Autodesk Inventor part; units mm, degrees
ref_plane "YZ Plane" through (0, 0, 0) normal (1, 0, 0) x (0, 1, 0)
ref_plane "XZ Plane" through (0, 0, 0) normal (0, 1, 0) x (-1, 0, 0)
ref_plane "XY Plane" through (0, 0, 0) normal (0, 0, 1) x (1, 0, 0)
sketch "Sketch1" plane through (0, 0, 0) normal (0, 0, 1) x (1, 0, 0)
  line L0 (0, 0) -> (110, 0)
  line L1 (110, 0) -> (110, 73)
  line L2 (110, 73) -> (0, 73)
  line L3 (6, 57) -> (50, 57)
  line L4 (50, 57) -> (50, 27)
  line L5 (6, 57) -> (0, 57)
  line L6 (0, 73) -> (0, 57)
  line L7 (0, 27) -> (0, 0)
  line L8 (0, 27) -> (50, 27)
  dimension "d0" = 110
  dimension "d2" = 16
  dimension "d19" = 57
  dimension "d22" = 50
  dimension "d66" = 30
extrude "Extrusion1" add sketch "Sketch1" along normal blind 6
sketch "Sketch2" plane through (0, 0, 6) normal (0, 0, 1) x (1, 0, 0)
  line L0 (105, 0) -> (105, 5)
  line L1 (105, 5) -> (5, 5)
  line L2 (5, 5) -> (5, 0)
  line L3 (0, 27) -> (0, 0)
  line L4 (0, 0) -> (110, 0)
  dimension "d13" = 100
  dimension "d14" = 5
  dimension "d15" = 5
extrude "Extrusion2" cut sketch "Sketch2" against normal blind 10
sketch "Sketch3" plane through (0, 0, 0) normal (0, 0, -1) x (-1, 0, 0)
  line L0 (-331.8351, -68) -> (-331.8351, 72) construction
  line L1 (218.6881, -67.4159) -> (-331.3119, -67.4159)
  line L2 (-331.8351, 72) -> (218.1649, 72)
  line L3 (-50.021, 72.5841) -> (-50.021, -67.4159)
  line L4 (-301.8351, 60.0199) -> (-301.8351, -95.3329) construction
  line L5 (-194.8351, 50.8275) -> (-194.8351, -92.5752) construction
  line L6 (-289.8351, 60.0199) -> (-289.8351, -99.0099) construction
  line L7 (-182.8351, -92.5752) -> (-182.8351, 81.6223) construction
  line L8 (-224.6619, -78.1083) -> (-224.6619, -12.2159) construction
  line L9 (-184.2519, -76.0321) -> (-184.2519, -10.2421) construction
  line L10 (-223.8335, -61.4159) -> (-147.922, -61.4159) construction
  line L11 (-179.8519, -67.4159) -> (-179.8519, -42.4159) construction
  line L12 (-229.1619, -42.4159) -> (-229.1619, -67.4159) construction
  line L13 (-73.021, 109.947) -> (-73.021, -118.6448) construction
  line L14 (-147.521, 95.654) -> (-147.521, -118.6448) construction
  line L15 (-208.521, 101.2387) -> (-208.521, -106.3335) construction
  line L16 (-237.7385, -71.614) -> (-237.7385, -46.614)
  line L17 (243.9615, -46.614) -> (243.9615, -71.614)
  line L18 (-92.021, 52) -> (-57.021, 52) construction
  line L19 (-57.021, 52) -> (-57.021, 27) construction
  line L20 (-57.021, 27) -> (-92.021, 27) construction
  line L21 (-92.021, 27) -> (-92.021, 52) construction
  line L22 (-301.8351, 2.5165) -> (201.7932, 2.5165) construction
  line L23 (-105, 0) -> (-105, 5)
  line L24 (-105, 5) -> (-5, 5)
  line L25 (-5, 5) -> (-5, 0)
  line L26 (0, 0) -> (-5, 0)
  line L27 (0, 27) -> (0, 0)
  line L28 (-50, 27) -> (0, 27)
  line L29 (-50, 57) -> (-50, 27)
  line L30 (0, 57) -> (-50, 57)
  line L31 (0, 73) -> (0, 57)
  line L32 (-110, 73) -> (0, 73)
  line L33 (-110, 0) -> (-110, 73)
  line L34 (-105, 0) -> (-110, 0)
  point P0 (-53.9258, 1.4801)
  point P1 (-331.3119, -67.4159)
  point P2 (-266.7948, -13.3199)
  point P3 (-301.8351, 60.0199)
  point P4 (-301.8351, -95.3329)
  point P5 (-289.8351, 2.5165)
  point P6 (-194.8351, 2.5165)
  point P7 (-182.8351, 2.5165)
  point P8 (189.7932, 2.5165)
  point P9 (94.7932, 2.5165)
  point P10 (82.7932, 2.5165)
  point P11 (-50.021, -58.9159)
  point P12 (-224.6619, -61.4159)
  point P13 (-184.2519, -61.4159)
  point P14 (124.6199, -61.4159)
  point P15 (84.2099, -61.4159)
  point P16 (-73.021, 12.3841)
  point P17 (-27.021, 12.3841)
  point P18 (-319.3351, 69)
  point P19 (-261.0351, 69)
  point P20 (-202.7351, 69)
  point P21 (-144.4351, 69)
  point P22 (-86.1351, 69)
  point P23 (-27.8351, 69)
  point P24 (30.4649, 69)
  point P25 (88.7649, 69)
  point P26 (147.0649, 69)
  point P27 (205.3649, 69)
  point P28 (-325.3351, 62)
  point P29 (-325.3351, 54)
  point P30 (-325.3351, 46)
  point P31 (-325.3351, 38)
  point P32 (-325.3351, 30)
  point P33 (-325.3351, 22)
  point P34 (-325.3351, 14)
  point P35 (-325.3351, 6)
  point P36 (-325.3351, -2)
  point P37 (-325.3351, -10)
  point P38 (-325.3351, -18)
  point P39 (-325.3351, -26)
  point P40 (-325.3351, -34)
  point P41 (225.2932, -34)
  point P42 (225.2932, -26)
  point P43 (225.2932, -18)
  point P44 (225.2932, -10)
  point P45 (225.2932, -2)
  point P46 (225.2932, 6)
  point P47 (225.2932, 14)
  point P48 (225.2932, 22)
  point P49 (225.2932, 30)
  point P50 (225.2932, 38)
  point P51 (225.2932, 46)
  point P52 (225.2932, 54)
  point P53 (225.2932, 62)
  point P54 (-242.2385, -65.614)
  point P55 (248.4615, -65.614)
  dimension "d32" = 30
  dimension "d33" = 12
  dimension "d34" = 137
  dimension "d35" = 12
  dimension "d36" = 8.5
  dimension "d37" = 4.4
  dimension "d38" = 4.5
  dimension "d39" = 6
  dimension "d40" = 23
  dimension "d41" = 97.5
  dimension "d42" = 158.5
  dimension "d43" = 3
  dimension "d44" = 12.5
  dimension "d45" = 58.3
  dimension "d46" = 6.5
  dimension "d47" = 10
  dimension "d48" = 8
  dimension "d49" = 35
  dimension "d50" = 35
  dimension "d51" = 25
  dimension "d52" = 4.5
  dimension "d53" = 4.5
  dimension "d56" = 20
  dimension "d57" = 7
  dimension "d58" = 1
hole "Hole1" at (50.021, -58.9159, 0) at (301.8351, 2.5165, 0) at (242.2385, -65.614, 0) at (194.8351, 2.5165, 0) at (289.8351, 2.5165, 0) at (182.8351, 2.5165, 0) at (-189.7932, 2.5165, 0) at (-201.7932, 2.5165, 0) at (-94.7932, 2.5165, 0) at (-82.7932, 2.5165, 0) at (224.6619, -61.4159, 0) at (184.2519, -61.4159, 0) at (-124.6199, -61.4159, 0) at (-84.2099, -61.4159, 0) at (73.021, 12.3841, 0) at (27.021, 12.3841, 0) at (325.3351, 62, 0) at (325.3351, 54, 0) at (325.3351, 46, 0) at (325.3351, 38, 0) at (325.3351, 30, 0) at (325.3351, 22, 0) at (325.3351, 14, 0) at (325.3351, 6, 0) at (325.3351, -2, 0) at (325.3351, -10, 0) at (325.3351, -18, 0) at (325.3351, -26, 0) at (325.3351, -34, 0) at (-225.2932, -34, 0) at (-225.2932, -26, 0) at (-225.2932, -18, 0) at (-225.2932, -10, 0) at (-225.2932, -2, 0) at (-225.2932, 6, 0) at (-225.2932, 14, 0) at (-225.2932, 22, 0) at (-225.2932, 30, 0) at (-225.2932, 38, 0) at (-225.2932, 46, 0) at (-225.2932, 54, 0) at (-225.2932, 62, 0) at (57.021, 52, 0) at (57.021, 27, 0) at (92.021, 27, 0) at (92.021, 52, 0) at (-248.4615, -65.614, 0) at (27.8351, 69, 0) at (86.1351, 69, 0) direction (0, 0, 1) diameter 1 end through all
properties part number "cerceau_front"
Source: CAD feature listing. Evaluate the final solid. Frame: model axes, mm. A direction names the side the tool comes from. Give positions to 0.01 mm unless a question says otherwise; leave off trailing zeros. Order: outer loops, then holes, each group sorted by start corner. A loop starts at its lowest first (then second) coordinate and runs counter-clockwise, first axis right, second up.
(1) Section query D-D (x = 80). Return the cut outline in (y, z), plus the area to 3 significant figures.
(2) Pull-direction query (Y, two-part tool) for faces 4 (the face through (56, 73, 3)), 5 (the face through (25, 57, 3)), 6 (the face through (56, 5, 3)), 7 (the face through (50, 42, 3)); classes: +Y half, -Y half, draft (parallel to the pull), parting line (faces both ways), or undercut.
(3) Contact query for a flat-ended pin moving along its axis: P1, Ø3, axis at x = 41.5, z = 4, coming from the -Y side. Output: stop coordinate, or through.
(4) Access query for faces 1 (the face through (25, 27, 3)), 2 (the face through (107, 0, 3)), 3 (the face through (105, 2, 3)). Directions: +Z, -Z, +X, -X, +Y, -Y. A direction counts if a zero-diameter tool reaches every point of the face in a straight line with its end or side. Return the directions, or none.
(5) Section query B-B (z = 5). State how many separate pieces and enclosed holes the cut face has, plus the area to 3 significant figures.
(6) Section query A-A (x = 36). Return the cut outline in (y, z), plus the area to 3 significant figures.
(7) Material intervals for line 1 along Y through (x, z) = (36.5, 0.65); line 2 along X through (y, z) = (4.5, 3.3); line 3 along Y through (x, z) = (86, 2.4), sorted ascending.
(8) Section query C-C (y = 33). Return the cut outline in (x, z), plus the area to 3 significant figures.
Outcome:
1. outline: (5, 0) - (73, 0) - (73, 6) - (5, 6) - close
1. area: 408 mm2
2. face 4: +Y half
2. face 5: undercut
2. face 6: -Y half
2. face 7: undercut
3. P1: stops at y = 5
4. face 1: +Z, -Z, -X
4. face 2: +Z, -Z, +X, -X, -Y
4. face 3: +Z, -Z, -Y
5. separate pieces: 1
5. enclosed holes: 8
5. area: 6,020 mm2
6. outline: (5, 0) - (27, 0) - (27, 6) - (5, 6) - close; (57, 0) - (73, 0) - (73, 6) - (57, 6) - close
6. area: 228 mm2
7. line 1: y = 5 to 27, 57 to 73
7. line 2: x = 0 to 5, 105 to 110
7. line 3: y = 5 to 68.52, 69.48 to 73
8. outline: (50, 0) - (110, 0) - (110, 6) - (50, 6) - close
8. area: 360 mm2
